from build123d import *


with BuildPart() as part:
    # 草图1 → 旋转3 (revolve)
    with BuildSketch(Plane.XY):
        with BuildLine():
            Line((-2, 0), (0, 0))
            Line((0, 0), (0, 4))
            ThreePointArc((0, 4), (-3.863703305, 1.03527618), (-2, -3.464101615))
            Line((-2, -3.464101615), (-2, 0))
        make_face()
        with BuildLine():
            Line((0, -4), (0, 0))
            Line((0, 0), (-2, 0))
            Line((-2, 0), (-2, -3.464101615))
            ThreePointArc((-2, -3.464101615), (-1.03527618, -3.863703305), (0, -4))
        make_face()
    revolve(axis=Axis((0, -4, 0), (0, -1, 0)))

    # 草图3 → 旋转4 (revolve)
    with BuildSketch(Plane.XY):
        with BuildLine():
            Line((0, -43), (0, -2))
            ThreePointArc((0, -2), (-1.414213562, -1.414213562), (-2, 0))
            Line((-2, 0), (-2, -2))
            Line((-2, -2), (-2, -43))
            Line((-2, -43), (0, -43))
        make_face()
    revolve(axis=Axis((0, -2, 0), (0, -1, 0)))

    # 草图4 → 旋转6 (revolve)
    with BuildSketch(Plane.XZ.offset(43)):
        with BuildLine():
            Line((-52.778814048, 0), (-4, 0))
            ThreePointArc((-4, 0), (-3.863703305, 1.03527618), (-3.464101615, 2))
            Line((-3.464101615, 2), (-52.778814048, 2))
            Line((-52.778814048, 2), (-52.778814048, 0))
        make_face()
        with BuildLine():
            Line((-4, 0), (-2, 0))
            ThreePointArc((-2, 0), (-1.414213562, 1.414213562), (0, 2))
            Line((0, 2), (-0.493950763, 2))
            Line((-0.493950763, 2), (-3.464101615, 2))
            ThreePointArc((-3.464101615, 2), (-3.863703305, 1.03527618), (-4, 0))
        make_face()
        with BuildLine():
            Line((0, 2), (0, 0))
            Line((0, 0), (2, 0))
            ThreePointArc((2, 0), (1.414213562, 1.414213562), (0, 2))
        make_face()
        with BuildLine():
            Line((-2, 0), (-0.493950763, 0))
            Line((-0.493950763, 0), (0, 0))
            Line((0, 0), (0, 2))
            ThreePointArc((0, 2), (-1.414213562, 1.414213562), (-2, 0))
        make_face()
    revolve(axis=Axis((-0.493950763, -43, 0), (-1, 0, 0)))


solid = part.part
Model file for the job. Use its own axes, mm. Give positions to 0.01 mm unless a question says otherwise; leave off trailing zeros. Order: outer loops, then holes, each group sorted by start corner. A loop starts at its lowest first (then second) coordinate and runs counter-clockwise, first axis right, second up. Notation, with made-up numbers: (24.5, 17) - (35.5, 17) arc R10 ccw to (35.5, 26) - close; hole circle Ø1 at (-38.5, 8.25). An arc over 180 degrees is marked (long way). Return JSON: item names as keys, results as strings.
1) Probe line 1 (Y direction, x = -22, z = -0.25); line 2 (Y direction, x = -33, z = -0.5); line 3 (X direction, y = -14.5, z = -0.5). List the from-to ranges inside material, lowest first. Write a range as from..to.
Geometry says:
{"line 1": "-44.98..-41.02", "line 2": "-44.94..-41.06", "line 3": "-1.94..1.94"}
2) Pull direction Y, two halves, no side cores. Call faces 1 (the flat face through (-52.779, -43, 0)), 2 (the cylindrical face through (-0.923, -23.509, 1.774)): pulls with the +Y half, pulls with the -Y half, needs draft (parallel to the pull), parting line crosses it, or undercut.
Geometry says:
{"face 1": "needs draft", "face 2": "undercut"}
3) Cut at B-B, the plane y = -19.5. Give the cut face in (x, z), plus the area to 3 significant figures.
Geometry says:
{"outline": "circle Ø4 at (0, 0)", "area": "12.6 mm²"}
4) Cut at C-C, the plane x = -9. Give the cut face in (y, z), plus the area to 3 significant figures.
Geometry says:
{"outline": "circle Ø4 at (-43, 0)", "area": "12.6 mm²"}
5) Cut at A-A, the plane z = 0. Give the cut face in (x, y).
Geometry says:
{"outline": "(-52.78, -45) - (0, -45) arc R2 ccw to (2, -43) - (2, -3.46) arc R4 ccw (long way) to (-2, -3.46) - (-2, -41) - (-52.78, -41) - close"}
